Drawing for the job (mm, zero at the part's lowest x, y, z). Coordinates: 2 decimals unless noted, no trailing zeros. Write each loop counter-clockwise with the first axis right and the second up, starting at its lowest first coordinate (ties: lowest second). Pieces come first, ordered by that corner, then holes. Notation, with made-up numbers: (44, -7) -> (91, -7) arc R18 cw to (91, 25) -> close; hole circle Ø1 at (46, -35.5). An arc over 180 degrees is marked (long way). Write each question's results on one line, items separated by ' | '. Start each with the question number.
Q1. Saw through at B-B on z = 58. Give the cut face in (x, y).
Q2. Saw through at A-A on y = 52.5. Give the cut face in (x, z).
Q3. Drill centre lines: line 1 (Z direction, x = 2.35, y = 35.5); line 2 (Z direction, x = 2.75, y = 55); line 3 (Y direction, x = 2.7, z = 12). Where is each one in solid material? Low to high.
Q4. Saw through at C-C on x = 0.5. Give the cut face in (y, z).
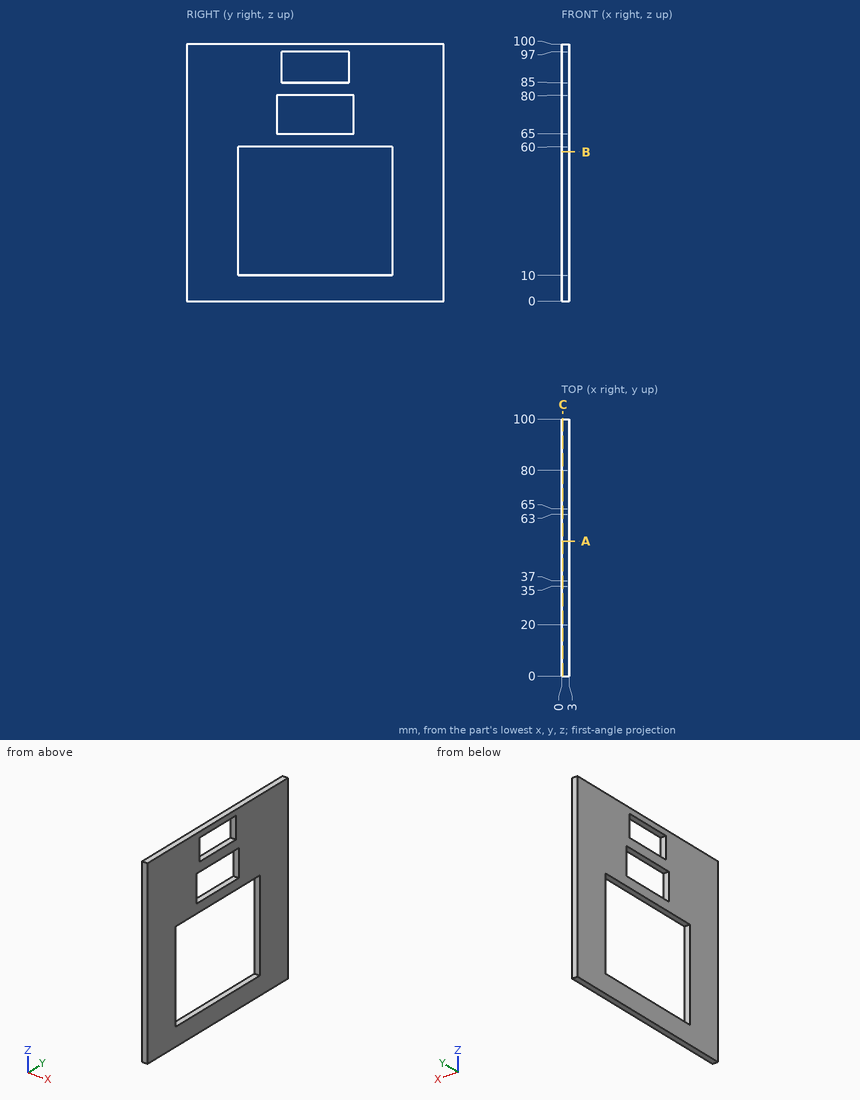
Returned:
1) outline: (0, 0) -> (3, 0) -> (3, 20) -> (0, 20) -> close; (0, 80) -> (3, 80) -> (3, 100) -> (0, 100) -> close
2) outline: (0, 0) -> (3, 0) -> (3, 10) -> (0, 10) -> close; (0, 60) -> (3, 60) -> (3, 65) -> (0, 65) -> close; (0, 80) -> (3, 80) -> (3, 85) -> (0, 85) -> close; (0, 97) -> (3, 97) -> (3, 100) -> (0, 100) -> close
3) line 1: z = 0 to 10, 60 to 65, 80 to 100 | line 2: z = 0 to 10, 60 to 65, 80 to 85, 97 to 100 | line 3: y = 0 to 20, 80 to 100
4) outline: (0, 0) -> (100, 0) -> (100, 100) -> (0, 100) -> close; hole (20, 10) -> (80, 10) -> (80, 60) -> (20, 60) -> close; hole (35, 65) -> (65, 65) -> (65, 80) -> (35, 80) -> close; hole (37, 85) -> (63, 85) -> (63, 97) -> (37, 97) -> close
